Geometry check sheet. Reference: drawing and pictorial views, mm from the part's lowest x, y, z. A direction names the side the tool comes from. Round coordinates to 2 decimals unless told otherwise and drop trailing zeros. Write each loop counter-clockwise with the first axis right and the second up, starting at its lowest first coordinate (ties: lowest second). Pieces come first, ordered by that corner, then holes. Notation, with made-up numbers: M 72,-22 L 102,-22 A9 cw 102,-6 Z; hole C -16,79.25 d7. An arc over 180 degrees is marked long. Answer in a Markdown table with one row per item.
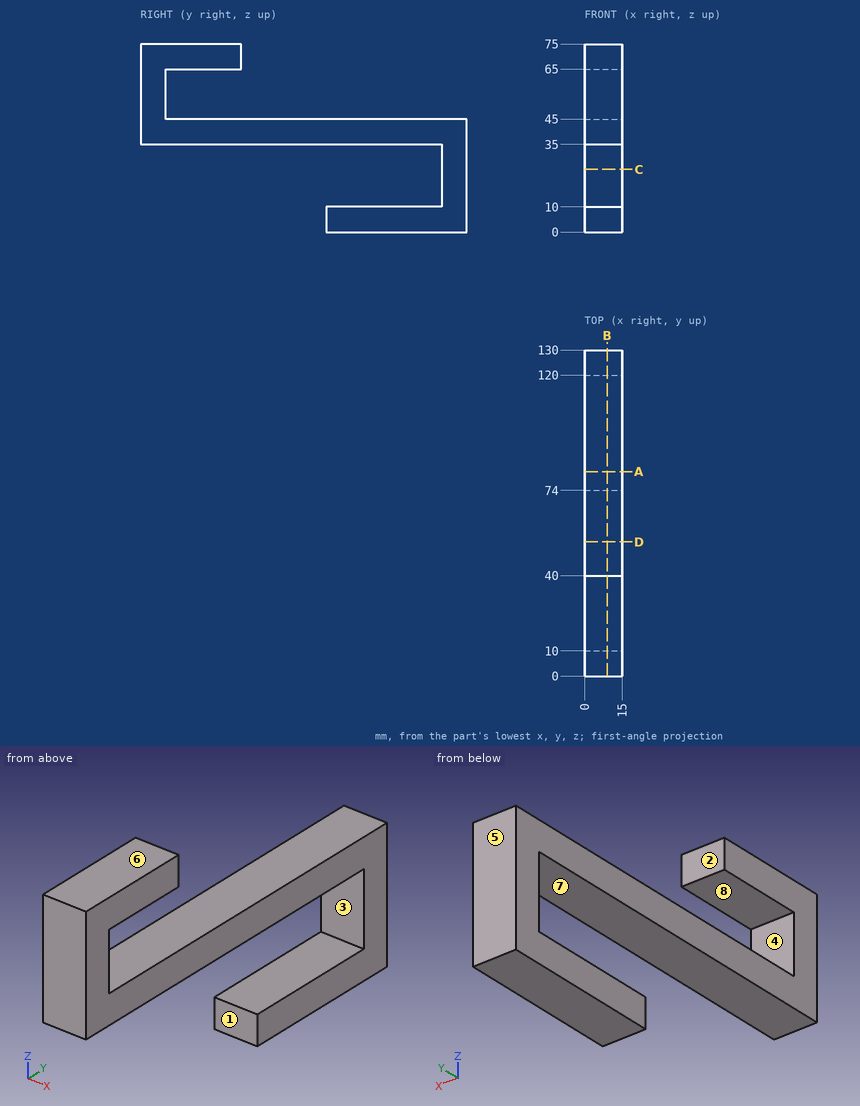
1. Section check A-A, the plane y = 81.5. Record the cut outline in (x, z).
Found:
| item | result |
|---|---|
| outline | M 0,0 L 15,0 L 15,10 L 0,10 Z; M 0,35 L 15,35 L 15,45 L 0,45 Z |
2. Draft check along Z on the marked faces 5, 6, 7 and 8. Enter one of: +Z half, -Z half, draft (parallel to the pull), parting line (faces both ways), or undercut.
Found:
| item | result |
|---|---|
| face 5 | draft |
| face 6 | +Z half |
| face 7 | undercut |
| face 8 | undercut |
3. Go/stop test with flat-tipped pins: pin 1 (8 mm diameter, centred on x = 4.5, z = 69.5, fed in from +Y); pin 2 (7.5 mm diameter, centred on x = 7, y = 106, fed in from +Z); pin 3 (4.5 mm diameter, centred on x = 4, z = 25.5, fed in from -Y). Record where each tip stops, or that it passes through.
Found:
| item | result |
|---|---|
| pin 1 | stops at y = 40 |
| pin 2 | stops at z = 45 |
| pin 3 | stops at y = 120 |
4. Section check C-C, the plane z = 25. Record the cut outline in (x, y), and give its area (3 significant figures).
Found:
| item | result |
|---|---|
| outline | M 0,120 L 15,120 L 15,130 L 0,130 Z |
| area | 150 mm2 |
5. Section check D-D, the plane y = 53.5. Record the cut outline in (x, z).
Found:
| item | result |
|---|---|
| outline | M 0,35 L 15,35 L 15,45 L 0,45 Z |
6. Access from +Z, -Z, +X, -X, +Y, -Y to the whole of each face (thin tool, end or side, straight path). Record for the marked faces 1, 2, 3 and 4.
Found:
| item | result |
|---|---|
| face 1 | -Z, +X, -X, -Y |
| face 2 | +Z, +X, -X, +Y |
| face 3 | +X, -X, -Y |
| face 4 | +X, -X, +Y |
7. Scan lines: L1, parallel to Z at x = 1.75, y = 87.5; L2, parallel to Z at x = 9, y = 35.5; L3, parallel to Y at x = 7.5, z = 52. Record each from-to range of solid material in increasing order.
Found:
| item | result |
|---|---|
| L1 | z = 0 to 10, 35 to 45 |
| L2 | z = 35 to 45, 65 to 75 |
| L3 | y = 0 to 10 |
8. Section check B-B, the plane x = 9. Record the cut outline in (y, z), and give its area (3 significant figures).
Found:
| item | result |
|---|---|
| outline | M 0,35 L 120,35 L 120,10 L 74,10 L 74,0 L 130,0 L 130,45 L 10,45 L 10,65 L 40,65 L 40,75 L 0,75 Z |
| area | 2,710 mm2 |
